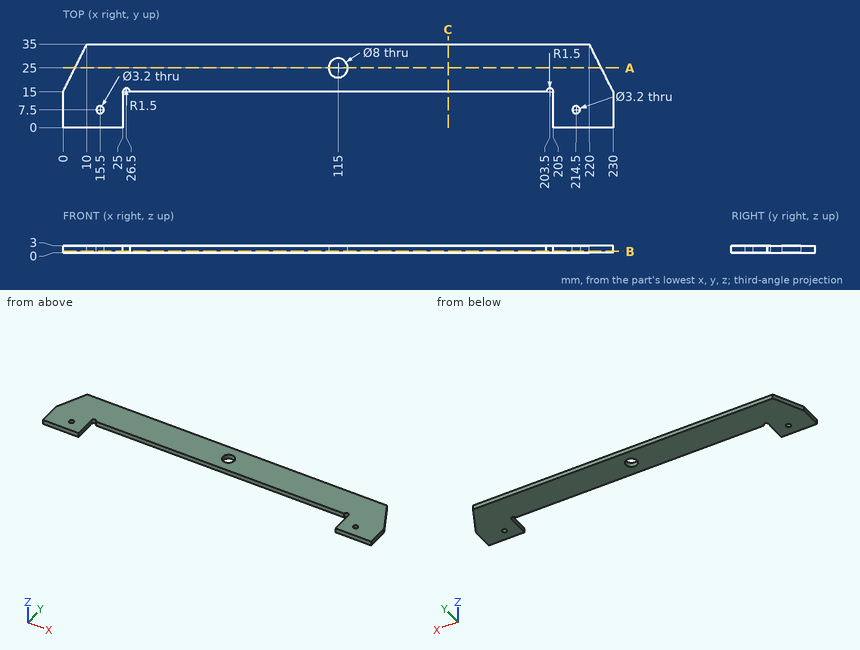
Verification items for this drawing (mm, ordinates from the low corner). Give positions to 0.01 mm unless a question says otherwise; leave off trailing zeros. Loops run counter-clockwise (first coordinate to the right, second up) from the corner with the lowest first, then second, coordinate; pieces in that order, holes last. Notation, with made-up numbers: (5.5, -17.5) - (23.5, -17.5) arc R25 ccw to (23.5, -5.5) - close; hole circle Ø1 at (13.25, 83). An arc over 180 degrees is marked (long way). Write item = value, one per line. Start each with the question number.
Q1. Thickness scan on line 1 (Y direction, x = 214.5, z = 1.9); line 2 (X direction, y = 4, z = 1.65); line 3 (Y direction, x = 100, z = 0.6). Record the ranges inside material, lowest first.
Q2. Cross-section at C-C, the plane x = 161. Enter the section's corners in (y, z).
Q3. Cross-section at B-B, the plane z = 0.6. Enter the section's corners in (x, y), and give its area (3 significant figures).
Q4. Cross-section at A-A, the plane y = 25. Enter the section's corners in (x, z), and give its area (3 significant figures).
Q5. Depth check by flat-ended pin: P1, Ø3, axis at x = 214.5, y = 7.5, coming from the +Z side; P2, Ø1.5, axis at x = 54.5, z = 1, coming from the -Y side. Enter the tip coordinate at first touch or a pass-through.
Answer key:
q1.line_1 = 0 to 5.9, 9.1 to 35
q1.line_2 = 0 to 25, 205 to 230
q1.line_3 = 15 to 35
q2.outline = (15, 0) - (35, 0) - (35, 3) - (15, 3) - close
q3.outline = (0, 0) - (25, 0) - (25, 15) arc R1.5 cw to (28, 15) - (202, 15) arc R1.5 cw to (205, 15) - (205, 0) - (230, 0) - (230, 15) - (220, 35) - (10, 35) - (0, 15) - close; hole circle Ø3.2 at (15.5, 7.5); hole circle Ø8 at (115, 25); hole circle Ø3.2 at (214.5, 7.5)
q3.area = 5,080 mm^2
q4.outline = (5, 0) - (111, 0) - (111, 3) - (5, 3) - close; (119, 0) - (225, 0) - (225, 3) - (119, 3) - close
q4.area = 636 mm^2
q5.P1 = through
q5.P2 = 15
